Build history of the part. All positions in model axes, mm. Face numbers are marked on the shaded views. A direction names the side the tool comes from. Round coordinates to 2 decimals unless told otherwise and drop trailing zeros. Order: outer loops, then holes, each group sorted by start corner. A loop starts at its lowest first (then second) coordinate and runs counter-clockwise, first axis right, second up. Notation, with made-up numbers: (-32, 15) -> (-14, 15) arc R23 cw to (-14, 36) -> close; hole circle Ø7 at (-28, 10.5). An arc over 180 degrees is marked (long way). Write item = value, one per line.
from build123d import *

# Parameters (mm, degrees)
SKETCH_1_R          = 12.5
EXTRUDE_1_DEPTH     = 57.5
SKETCH_2_R          = 3.5
EXTRUDE_2_DEPTH     = 2.5
SKETCH_3_R          = 2
EXTRUDE_3_DEPTH     = 9.5
CUT_EXTRUDE_1_DEPTH = 8
SKETCH_5_R          = 1.5
CUT_EXTRUDE_2_DEPTH = 5


with BuildPart() as part:
    # 草图1 → 凸台-拉伸1 (new body)
    with BuildSketch(Plane(origin=(0, 0, 0), x_dir=(1, 0, 0), z_dir=(0, 1, 0))):
        with Locations(Location((0, 0, 0), (0, 0, 270))):
            Circle(SKETCH_1_R)
    extrude(amount=EXTRUDE_1_DEPTH)

    # 草图2 → 凸台-拉伸2 (add)
    with BuildSketch(Plane(origin=(0, 57.5, 0), x_dir=(1, 0, 0), z_dir=(0, 1, 0))):
        with Locations(Location((0, 0, 0), (0, 0, 270))):
            Circle(SKETCH_2_R)
    extrude(amount=EXTRUDE_2_DEPTH)

    # 草图3 → 凸台-拉伸3 (add)
    with BuildSketch(Plane(origin=(0, 60, 0), x_dir=(1, 0, 0), z_dir=(0, 1, 0))):
        with Locations(Location((0, 0, 0), (0, 0, 270))):
            Circle(SKETCH_3_R)
    extrude(amount=EXTRUDE_3_DEPTH)

    # 草图4 → 切除-拉伸1 (cut)
    with BuildSketch(Plane(origin=(0, 69.5, 0), x_dir=(1, 0, 0), z_dir=(0, 1, 0))):
        Polygon((-50.671161076, 1.5), (-1.322875656, 1.5), (1.322875656, 1.5), (50.671161076, 1.5), (50.671161076, 100.196570842), (-50.671161076, 100.196570842), align=None)
    extrude(amount=-CUT_EXTRUDE_1_DEPTH, mode=Mode.SUBTRACT)

    # 草图5 → 切除-拉伸2 (cut)
    with BuildSketch(Plane(origin=(0, 57.5, 0), x_dir=(1, 0, 0), z_dir=(0, 1, 0))):
        with Locations(Location((0, 8.5, 0), (0, 0, 270))):
            Circle(SKETCH_5_R)
        with Locations(Location((0, -8.5, 0), (0, 0, 270))):
            Circle(SKETCH_5_R)
    extrude(amount=-CUT_EXTRUDE_2_DEPTH, mode=Mode.SUBTRACT)


solid = part.part
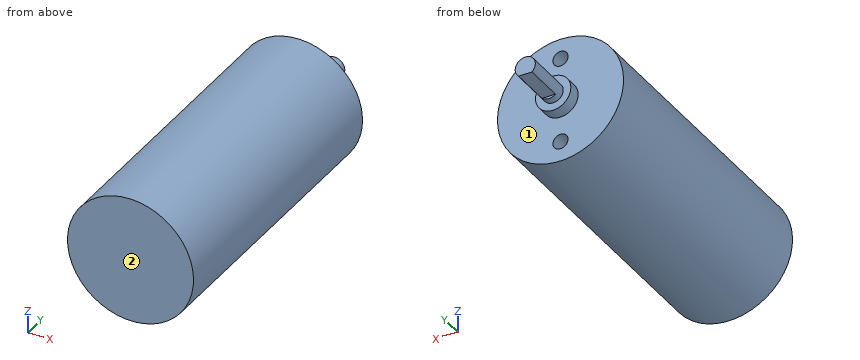
Q1. Cut at A-A, the plane x = 0. List the corners of the cut face in (y, z), and give its area (3 significant figures).
Check values:
outline = (0, -12.5) -> (57.5, -12.5) -> (57.5, -10) -> (52.5, -10) -> (52.5, -7) -> (57.5, -7) -> (57.5, -3.5) -> (60, -3.5) -> (60, -2) -> (61.5, -2) -> (61.5, -1.5) -> (69.5, -1.5) -> (69.5, 2) -> (60, 2) -> (60, 3.5) -> (57.5, 3.5) -> (57.5, 7) -> (52.5, 7) -> (52.5, 10) -> (57.5, 10) -> (57.5, 12.5) -> (0, 12.5) -> close
area = 1,460 mm²
Q2. Probe probe 1 along Y at (x, z) = (5, -5.25); probe 2 along X at (y, z) = (53.5, -8.25); probe 3 along Z at (x, y) = (-0.25, 3.5). List the from-to ranges inside material, lowest first.
Check values:
probe_1 = 0 to 57.5
probe_2 = -9.39 to -1.48, 1.48 to 9.39
probe_3 = -12.5 to 12.5
Q3. Cut at C-C, the plane y = 14.5. List the corners of the cut face in (x, z), and give its area (3 significant figures).
Check values:
outline = circle Ø25 at (0, 0)
area = 491 mm²
Q4. Flat gauge pins, fed straight in: pin 1 (2.5 mm diameter, centred on x = 0, z = -8.5, fed in from +Y); pin 2 (6 mm diameter, centred on y = 57.5, z = -7.5, fed in from +X); pin 3 (1.3 mm diameter, centred on x = -0.5, y = 65, fed in from -Z). Where does each tip first touch, or does it go through?
Check values:
pin_1 = 52.5
pin_2 = 11.66
pin_3 = -1.5
Q5. Cut at B-B, the plane z = 0. List the corners of the cut face in (x, y), and give its area (3 significant figures).
Check values:
outline = (-12.5, 0) -> (12.5, 0) -> (12.5, 57.5) -> (3.5, 57.5) -> (3.5, 60) -> (2, 60) -> (2, 69.5) -> (-2, 69.5) -> (-2, 60) -> (-3.5, 60) -> (-3.5, 57.5) -> (-12.5, 57.5) -> close
area = 1,490 mm²
Q6. Which spindle directions (+Z, -Z, +X, -X, +Y, -Y) get a long thin tool onto all of the face, cutting with end or side? Do the marked faces 1 and 2. Say none if no direction does.
Check values:
face_1 = +Y
face_2 = +Z, -Z, +X, -X, -Y
Q7. Cut at D-D, the plane z = -8.5. List the corners of the cut face in (x, y).
Check values:
outline = (-9.17, 0) -> (9.17, 0) -> (9.17, 57.5) -> (1.5, 57.5) -> (1.5, 52.5) -> (-1.5, 52.5) -> (-1.5, 57.5) -> (-9.17, 57.5) -> close
